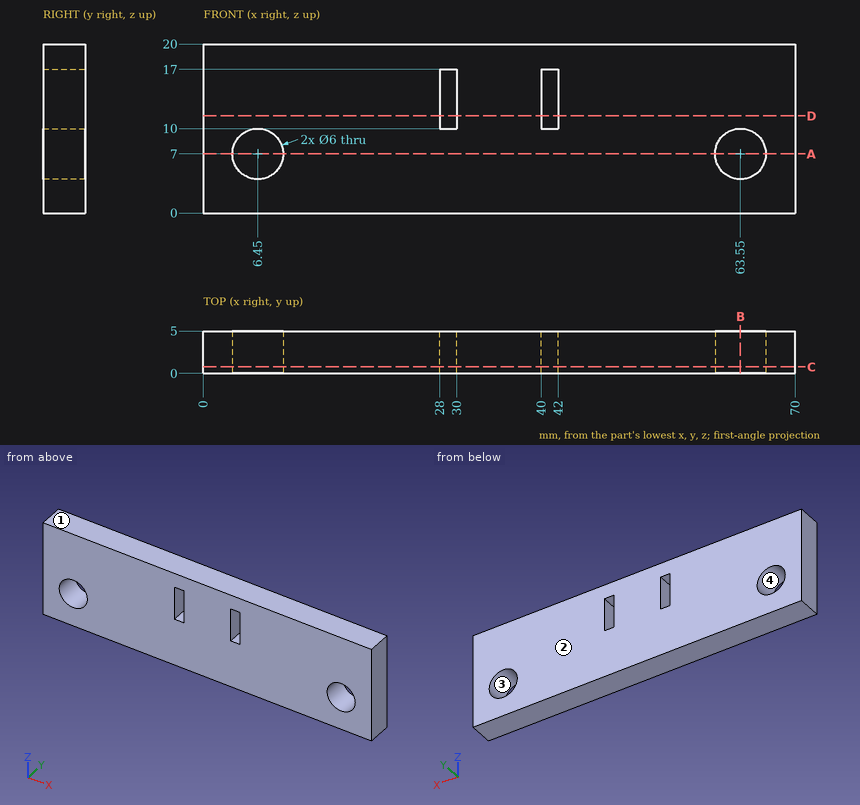
Answer from the drawing. Dimensions are ordinates in mm from the lowest x, y and z of the part. Coordinates: 2 decimals unless noted, no trailing zeros. Order: outer loops, then holes, each group sorted by start corner. A loop starts at its lowest first (then second) coordinate and runs counter-clockwise, first axis right, second up. Notation, with made-up numbers: (24, -23) -> (47, -23) arc R17 ccw to (47, -13) -> close; hole circle Ø10 at (-27, 85.25). An arc over 180 degrees is marked (long way). Answer as a JSON object with one key per item and string values.
1) This flat-tipped pin is pushed along its axis until it touches: pin 1 (5 mm diameter, centred on x = 6.45, z = 7, fed in from +Y). Where does it stop, or does it pass through?
Model answer:
{"pin 1": "passes through"}
2) Consider line 1 along X through (y, z) = (2.2, 7.25); line 2 along X through (y, z) = (0.6, 14); line 3 along Z through (x, y) = (41, 1.3). Determine where each line is inside the solid, lowest interval first. Write a range as from..to.
Model answer:
{"line 1": "x = 0..3.46, 9.44..60.56, 66.54..70", "line 2": "x = 0..28, 30..40, 42..70", "line 3": "z = 0..10, 17..20"}
3) A cutting plane is placed at D-D, the plane z = 11.5. Determine the outline of the cut face in (x, y).
Model answer:
{"outline": "(0, 0) -> (28, 0) -> (28, 5) -> (0, 5) -> close; (30, 0) -> (40, 0) -> (40, 5) -> (30, 5) -> close; (42, 0) -> (70, 0) -> (70, 5) -> (42, 5) -> close"}
4) The mould has two halves that part along Z. Classify the marked faces 1, 2, 3 and 4: released by +Z, released by -Z, zero draft, split by the parting line, or undercut.
Model answer:
{"face 1": "released by +Z", "face 2": "zero draft", "face 3": "undercut", "face 4": "undercut"}
5) A cutting plane is placed at B-B, the plane x = 63.55. Determine the outline of the cut face in (y, z).
Model answer:
{"outline": "(0, 0) -> (5, 0) -> (5, 4) -> (0, 4) -> close; (0, 10) -> (5, 10) -> (5, 20) -> (0, 20) -> close"}
6) A cutting plane is placed at A-A, the plane z = 7. Determine the outline of the cut face in (x, y).
Model answer:
{"outline": "(0, 0) -> (3.45, 0) -> (3.45, 5) -> (0, 5) -> close; (9.45, 0) -> (60.55, 0) -> (60.55, 5) -> (9.45, 5) -> close; (66.55, 0) -> (70, 0) -> (70, 5) -> (66.55, 5) -> close"}
7) A cutting plane is placed at C-C, the plane y = 0.75. Determine the outline of the cut face in (x, z).
Model answer:
{"outline": "(0, 0) -> (70, 0) -> (70, 20) -> (0, 20) -> close; hole circle Ø6 at (6.45, 7); hole (28, 10) -> (30, 10) -> (30, 17) -> (28, 17) -> close; hole (40, 10) -> (42, 10) -> (42, 17) -> (40, 17) -> close; hole circle Ø6 at (63.55, 7)"}
